```python
from build123d import *

# Parameters (mm, degrees)
SKETCH1_R           = 1.65
BOSS_EXTRUDE1_DEPTH = 2.5
SKETCH5_R           = 1.65
BOSS_EXTRUDE2_DEPTH = 1.5
CUT_EXTRUDE3_DEPTH  = 1


with BuildPart() as part:
    # Sketch1 → Boss-Extrude1 (new body)
    with BuildSketch(Plane.XY):
        with BuildLine():
            Line((-8.004553297, 23.25769142), (12, 23.25769142))
            Line((12, 23.25769142), (12, 0))
            Line((12, 0), (12, -2))
            Line((12, -2), (0.775731814, -2))
            Line((0.775731814, -2), (0.775731814, 0))
            Line((0.775731814, 0), (0.775731814, 3.25769142))
            Line((0.775731814, 3.25769142), (-13.882660061, 3.25769142))
            ThreePointArc((-13.882660061, 3.25769142), (-12.382699641, 13.680648524), (-8.004553297, 23.25769142))
        make_face()
        with Locations((6.74921921, 19.306101501)):
            Circle(SKETCH1_R, mode=Mode.SUBTRACT)
        with Locations((6.74921921, 1.806101501)):
            Circle(SKETCH1_R, mode=Mode.SUBTRACT)
    extrude(amount=BOSS_EXTRUDE1_DEPTH)

    # Sketch5 → Boss-Extrude2 (add)
    with BuildSketch(Plane.XY.offset(2.5)):
        Polygon((0.775731814, 3.25769142), (0.775731814, 23.25769142), (12, 23.25769142), (12, -2), (0.775731814, -2), align=None)
        with Locations((6.74921921, 19.306101501)):
            Circle(SKETCH5_R, mode=Mode.SUBTRACT)
        with Locations((6.74921921, 1.806101501)):
            Circle(SKETCH5_R, mode=Mode.SUBTRACT)
    extrude(amount=BOSS_EXTRUDE2_DEPTH)

    # Sketch6 → Cut-Extrude3 (cut)
    with BuildSketch(Plane(origin=(0, 0, 0), x_dir=(-1, 0, 0), z_dir=(0, 0, -1))):
        Polygon((-12, 23.25769142), (-12, -2), (-0.775731814, -2), (-0.775731814, 3.25769142), (2.826661011, 3.25769142), (2.826661011, 23.25769142), align=None)
    extrude(amount=-CUT_EXTRUDE3_DEPTH, mode=Mode.SUBTRACT)


solid = part.part
```
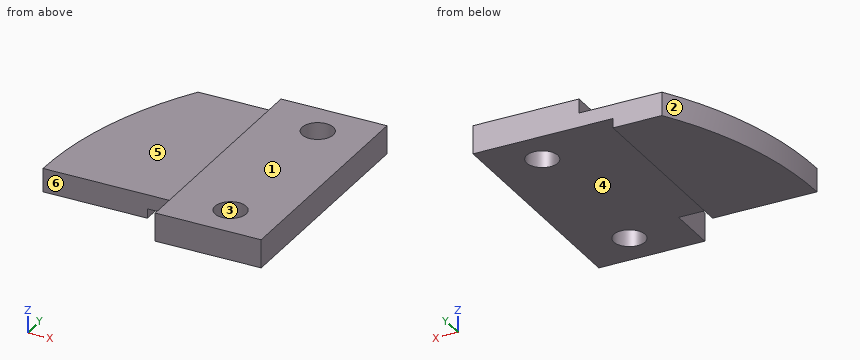
The listing builds one solid part. Answer for the finished solid, in the listing's coordinates (mm). Face numbers are marked on the shaded views. A direction names the side the tool comes from. Give positions to 0.01 mm unless a question says otherwise; leave off trailing zeros. Write each loop counter-clockwise with the first axis right and the second up, starting at its lowest first coordinate (ties: lowest second). Pieces come first, ordered by that corner, then holes. Notation, with made-up numbers: M 18,61.25 L 49,61.25 A32 ccw 49,89.25 Z; hole C -38,62.5 d6. An arc over 180 degrees is marked long. Write each question's results on one line, items separated by ' | '.
Q1. Flat-ended cylindrical pins translate along their axes: P1, Ø4.5, axis at x = 2, y = 11.5, coming from the -Z side; P2, Ø8, axis at x = -9.5, y = 4.5, coming from the +Z side; P3, Ø2, axis at x = -6, z = 1, coming from the -Y side. Find the tip coordinate at first contact, or state that the pin passes through.
Output values:
P1: z = 1 | P2: z = 2.5 | P3: y = 3.26
Q2. A tool of negligible diameter and unlimited length cuts with its end or side. For the marked faces 4, 5 and 6, from which of +Z, -Z, +X, -X, +Y, -Y can it reach the whole face along a straight path? Write none if from no direction.
Output values:
face 4: -Z, +X, +Y, -Y | face 5: +Z, -X, +Y, -Y | face 6: +Z, -Z, -X, -Y
Q3. Section A-A, the plane y = 18.25 is taken. Write down the section's boundary in (x, z), then the cut area to 3 significant figures.
Output values:
outline: M -10.71,0 L -2.83,0 L -2.83,1 L 5.48,1 L 5.48,4 L 0.78,4 L 0.78,2.5 L -10.71,2.5 Z; M 8.02,1 L 12,1 L 12,4 L 8.02,4 Z | area: 51.2 mm2
Q4. For a pull along X with two mould halves and no side action, classify the marked faces 1, 2 and 3 as released by +X, released by -X, zero draft, split by the parting line, or undercut.
Output values:
face 1: zero draft | face 2: released by -X | face 3: undercut
Q5. Consider L1, parallel to Y at x = 7, z = 2.25; L2, parallel to Z at x = 8.5, y = 21.25; L3, parallel to Z at x = -12.5, y = 8.25. Determine where each line is inside the solid, lowest interval first. Write a range as from..to.
Output values:
L1: -2..0.18, 3.44..17.68, 20.94..23.26 | L2: 1..4 | L3: 0..2.5
Q6. Section D-D, the plane y = 7.25 is taken. Write down the section's boundary in (x, z), then the cut area to 3 significant figures.
Output values:
outline: M -13.67,0 L -2.83,0 L -2.83,1 L 12,1 L 12,4 L 0.78,4 L 0.78,2.5 L -13.67,2.5 Z | area: 66.2 mm2
Q7. Section C-C, the plane x = -4 is taken. Write down the section's boundary in (y, z).
Output values:
outline: M 3.26,0 L 23.26,0 L 23.26,2.5 L 3.26,2.5 Z
Q8. Section B-B, the plane z = 1.45 is taken. Write down the section's boundary in (x, y), then the cut area to 3 significant figures.
Output values:
outline: M -13.88,3.26 L 0.78,3.26 L 0.78,-2 L 12,-2 L 12,23.26 L -8,23.26 A36.96 ccw Z; hole C 6.75,1.81 d3.3; hole C 6.75,19.31 d3.3 | area: 522 mm2
